Geometry check sheet. Reference: the model listing, model coordinates, mm. A direction names the side the tool comes from. Round coordinates to 2 decimals unless told otherwise and drop trailing zeros. Write each loop counter-clockwise with the first axis right and the second up, starting at its lowest first coordinate (ties: lowest second). Pieces come first, ordered by that corner, then holes. Notation, with made-up numbers: (65, -8.75) - (99, -8.75) arc R26 ccw to (99, 11.25) - close; hole circle Ø6 at (-7.5, 74.25). An arc over 180 degrees is marked (long way). Return JSON: item names as keys, results as strings. Group by question number.
from build123d import *

# Parameters (mm, degrees)
SKETCH1_W                                     = 17.5
SKETCH1_H                                     = 10
BASE_FLANGE1_DEPTH                            = 2
EDGE_FLANGE1_DEPTH                            = 17.5
EDGE_FLANGE2_STRIP_W                          = 9.4732
EDGE_FLANGE2_STRIP_H                          = 2
EDGE_FLANGE2_STRIP_CUT_DEPTH                  = 17.5
EDGE_FLANGE2_DEPTH                            = 17.5
EDGE_FLANGE3_STRIP_W                          = 9.4732
EDGE_FLANGE3_STRIP_H                          = 2
EDGE_FLANGE3_STRIP_CUT_DEPTH                  = 17.5
EDGE_FLANGE3_DEPTH                            = 17.5
SKETCH18_R                                    = 4
CUT_EXTRUDE2_DEPTH                            = 2
CSK_FOR_4_FLAT_HEAD_SOCKET_CAP_SCREW1_A_COUNT = 2
CSK_FOR_4_FLAT_HEAD_SOCKET_CAP_SCREW1_A_PITCH = 9.5
CUT_EXTRUDE3_DEPTH                            = 2


# Sheet-metal steps are written as plain solids
with BuildPart() as part:
    # Sketch1 → Base-Flange1 (new body)
    with BuildSketch(Plane(origin=(0, 0, 0), x_dir=(1, 0, 0), z_dir=(0, 1, 0))):
        Rectangle(SKETCH1_W, SKETCH1_H)
    extrude(amount=BASE_FLANGE1_DEPTH)

    # Edge-Flange1 section (across the edge) → Edge-Flange1 (add)
    with BuildSketch(Plane(origin=(-8.75, 2, 5.7366), x_dir=(0, 0, -1), z_dir=(1, 0, 0))):
        with BuildLine():
            Line((-2, 0.7366), (-2, 65.5))
            Line((-2, 65.5), (0, 65.5))
            Line((0, 65.5), (0, 0.7366))
            ThreePointArc((0, 0.7366), (0.215745145, 0.215745145), (0.7366, 0))
            Line((0.7366, 0), (0.7366, -2))
            ThreePointArc((0.7366, -2), (-1.198468417, -1.198468417), (-2, 0.7366))
        make_face()
    extrude(amount=EDGE_FLANGE1_DEPTH)

    # Edge-Flange2 strip (across the edge) → Edge-Flange2 strip cut (cut)
    with BuildSketch(Plane(origin=(-8.75, 67.5, 5.7366), x_dir=(0, -1, 0), z_dir=(1, 0, 0))):
        with Locations((-2, -1)):
            Rectangle(EDGE_FLANGE2_STRIP_W, EDGE_FLANGE2_STRIP_H)
    extrude(amount=EDGE_FLANGE2_STRIP_CUT_DEPTH, mode=Mode.SUBTRACT)

    # Edge-Flange2 section (across the edge) → Edge-Flange2 (add)
    with BuildSketch(Plane(origin=(-8.75, 67.5, 5.7366), x_dir=(0, -1, 0), z_dir=(1, 0, 0))):
        with BuildLine():
            Line((0, 0.7366), (0, 145.22348749))
            Line((0, 145.22348749), (2, 145.22348749))
            Line((2, 145.22348749), (2, 0.7366))
            ThreePointArc((2, 0.7366), (2.215745145, 0.215745145), (2.7366, 0))
            Line((2.7366, 0), (2.7366, -2))
            ThreePointArc((2.7366, -2), (0.801531583, -1.198468417), (0, 0.7366))
        make_face()
    extrude(amount=EDGE_FLANGE2_DEPTH)

    # Edge-Flange3 strip (across the edge) → Edge-Flange3 strip cut (cut)
    with BuildSketch(Plane(origin=(-8.75, 65.5, -139.48688749), x_dir=(0, 0, 1), z_dir=(1, 0, 0))):
        with Locations((-2, -1)):
            Rectangle(EDGE_FLANGE3_STRIP_W, EDGE_FLANGE3_STRIP_H)
    extrude(amount=EDGE_FLANGE3_STRIP_CUT_DEPTH, mode=Mode.SUBTRACT)

    # Edge-Flange3 section (across the edge) → Edge-Flange3 (add)
    with BuildSketch(Plane(origin=(-8.75, 65.5, -139.48688749), x_dir=(0, 0, 1), z_dir=(1, 0, 0))):
        with BuildLine():
            Line((0, 0.7366), (0, 16))
            Line((0, 16), (2, 16))
            Line((2, 16), (2, 0.7366))
            ThreePointArc((2, 0.7366), (2.215745145, 0.215745145), (2.7366, 0))
            Line((2.7366, 0), (2.7366, -2))
            ThreePointArc((2.7366, -2), (0.801531583, -1.198468417), (0, 0.7366))
        make_face()
    extrude(amount=EDGE_FLANGE3_DEPTH)

    # Sketch18 → Cut-Extrude2 (cut)
    with BuildSketch(Plane(origin=(0, 0, -139.48688749), x_dir=(-1, 0, 0), z_dir=(0, 0, -1))):
        with Locations(Location((0, 57.2634, 0), (0, 0, 90))):
            Circle(SKETCH18_R)
    extrude(amount=-CUT_EXTRUDE2_DEPTH, mode=Mode.SUBTRACT)

    # Sketch20 → CSK for #4 Flat Head Socket Cap Screw1 (revolve, cut)
    with BuildSketch(Plane(origin=(4.75, 0, 0), x_dir=(0, 0, -1), z_dir=(1, 0, 0))):
        Polygon((0, 0), (0, 2.980574487), (1.63195, 2), (1.63195, 1.848124365), (3.2385, 0), align=None)
    csk_for_4_flat_head_socket_cap_screw1 = revolve(axis=Axis((4.75, -6.35, 0), (0, 1, 0)), mode=Mode.SUBTRACT)

    # CSK for #4 Flat Head Socket Cap Screw1 a: CSK for #4 Flat Head Socket Cap Screw1 ×2
    with Locations(*[(-i * CSK_FOR_4_FLAT_HEAD_SOCKET_CAP_SCREW1_A_PITCH, 0, 0) for i in range(1, CSK_FOR_4_FLAT_HEAD_SOCKET_CAP_SCREW1_A_COUNT)]):
        add(csk_for_4_flat_head_socket_cap_screw1, mode=Mode.SUBTRACT)

    # Sketch23 → Cut-Extrude3 (cut)
    with BuildSketch(Plane.XZ.offset(-65.5)):
        with BuildLine():
            Line((-1.65, -119.25028749), (-1.65, -114.25028749))
            ThreePointArc((-1.65, -114.25028749), (0, -112.60028749), (1.65, -114.25028749))
            Line((1.65, -114.25028749), (1.65, -119.25028749))
            ThreePointArc((1.65, -119.25028749), (0, -120.90028749), (-1.65, -119.25028749))
        make_face()
    extrude(amount=-CUT_EXTRUDE3_DEPTH, mode=Mode.SUBTRACT)


solid = part.part
1. Section check A-A (z = 0). Enter the section's corners in (x, y).
2. Tool access check on faces 4 (the face through (-2.1, 53.6, -137.487)), 5 (the face through (0, 2, 0)), 6 (the face through (-1.53, 60.96, -138.5)), 7 (the face through (0, 34, 5.737)). Record the directions out of +Z, -Z, +X, -X, +Y, -Y that give a thin tool (end or side, any length) a straight path to the whole face; none if there is none.
3. Section check B-B (x = 0). Enter the section's corners in (y, z).
4. Depth check by flat-ended pin: pin 1 Ø6 at (x, z) = (2, -94.5) entering from -Y; pin 2 Ø1 at (x, z) = (-2.5, -139) entering from -Y; pin 3 Ø1.6 at (x, y) = (-3.5, 1) entering from -Z. Enter the tip coordinate at first touch or a pass-through.
5. Material ranges on line 1 along X through (y, z) = (1.9, 0); line 2 along Z through (x, y) = (2.75, 54); line 3 along Z through (x, y) = (8, 5), recorded low to high.
6. Section check C-C (y = 14.5). Enter the section's corners in (x, z).
7. Mould release check, pull along Z, two halves, no side actions. Record for faces 1 (the face through (-0.123, 66.72, -138.664)), 2 (the face through (-8.75, 66, -60)), 3 (the face through (6.44, 1.73, 0.38)): pulls with the +Z half, pulls with the -Z half, needs draft (parallel to the pull), parting line crosses it, or undercut.
Result sheet:
{
 "1": {"outline": "(-8.75, 0) - (-7.99, 0) - (-6.38, 1.85) - (-6.38, 2) - (-8.75, 2) - close; (-8.75, 65.5) - (8.75, 65.5) - (8.75, 67.5) - (-8.75, 67.5) - close; (-3.12, 1.85) - (-1.51, 0) - (1.51, 0) - (3.12, 1.85) - (3.12, 2) - (-3.12, 2) - close; (6.38, 1.85) - (7.99, 0) - (8.75, 0) - (8.75, 2) - (6.38, 2) - close"},
 "2": {"face 4": "+X, -X, -Y", "face 5": "-Z, +X, -X", "face 6": "-Z", "face 7": "+X, -X"},
 "3": {"outline": "(0, -5) - (2, -5) - (2, 5) arc R0.74 cw to (2.74, 5.74) - (64.76, 5.74) arc R0.74 cw to (65.5, 5) - (65.5, -112.6) - (67.5, -112.6) - (67.5, 5) arc R2.74 ccw to (64.76, 7.74) - (2.74, 7.74) arc R2.74 ccw to (0, 5) - close; (49.5, -139.49) - (53.26, -139.49) - (53.26, -137.49) - (49.5, -137.49) - close; (61.26, -139.49) - (64.76, -139.49) arc R2.74 ccw to (67.5, -136.75) - (67.5, -120.9) - (65.5, -120.9) - (65.5, -136.75) arc R0.74 cw to (64.76, -137.49) - (61.26, -137.49) - close"},
 "4": {"pin 1": "stops at y = 65.5", "pin 2": "stops at y = 49.5", "pin 3": "stops at z = -5"},
 "5": {"line 1": "x = -8.75 to -6.38, -3.12 to 3.12, 6.38 to 8.75", "line 2": "z = -139.49 to -137.49, 5.74 to 7.74", "line 3": "z = 5.74 to 7.74"},
 "6": {"outline": "(-8.75, 5.74) - (8.75, 5.74) - (8.75, 7.74) - (-8.75, 7.74) - close"},
 "7": {"face 1": "pulls with the -Z half", "face 2": "needs draft", "face 3": "undercut"}
}
